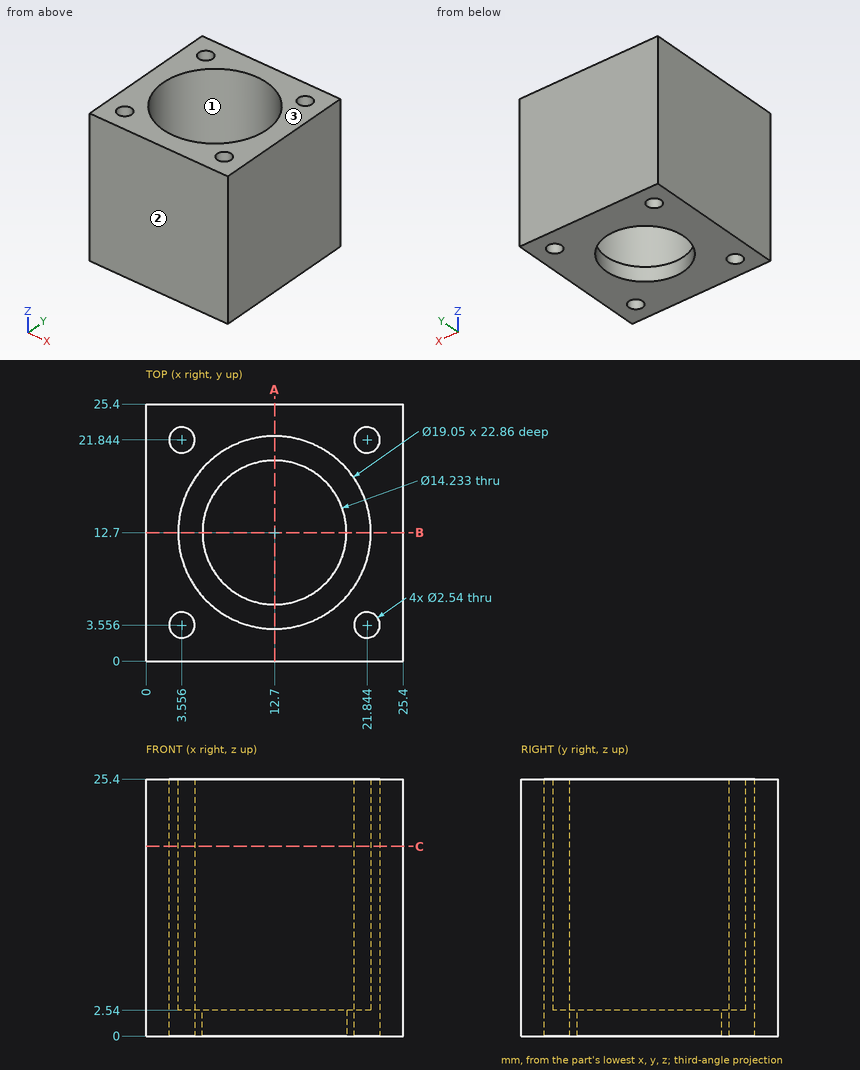
Check sheet for the drawn part. Datum: minimum x, y, z corner. Units: mm. Round coordinates to 2 decimals unless told otherwise and drop trailing zeros. Order: outer loops, then holes, each group sorted by start corner. A loop starts at its lowest first (then second) coordinate and runs counter-clockwise, first axis right, second up.
(1) Cross-section at A-A, the plane x = 12.7. Enter the section's corners in (y, z) (1 decimal).
(2) Draft check along Y on the marked faces 1, 2 and 3. Enter one of: pulls with the +Y half, pulls with the -Y half, needs draft (parallel to the pull), parting line crosses it, or undercut.
(3) Scan lines: probe 1 along X at (y, z) = (20.75, 18.5); probe 2 along Y at (x, z) = (12.7, 7.5) (3 decimals); probe 3 along Y at (x, z) = (21, 17.5) (3 decimals). Record each from-to range of solid material in increasing order.
(4) Cross-section at C-C, the plane z = 18.75. Enter the section's corners in (x, y) (3 decimals), and give its area (3 significant figures).
(5) Go/stop test with flat-tipped pins: P1, Ø15, axis at x = 12.7, y = 12.7, coming from the +Z side; P2, Ø1.5, axis at x = 3.556, y = 3.556, coming from the -Z side. Record where each tip stops, or that it passes through.
Check sheet entries:
1. outline: (0, 0) - (5.6, 0) - (5.6, 2.5) - (3.2, 2.5) - (3.2, 25.4) - (0, 25.4) - close; (19.8, 0) - (25.4, 0) - (25.4, 25.4) - (22.2, 25.4) - (22.2, 2.5) - (19.8, 2.5) - close
2. face 1: undercut
2. face 2: pulls with the -Y half
2. face 3: needs draft
3. probe 1: x = 0 to 2.91, 4.2 to 7.61, 17.79 to 21.2, 22.49 to 25.4
3. probe 2: y = 0 to 3.175, 22.225 to 25.4
3. probe 3: y = 0 to 2.607, 4.505 to 8.027, 17.373 to 20.895, 22.793 to 25.4
4. outline: (0, 0) - (25.4, 0) - (25.4, 25.4) - (0, 25.4) - close; hole circle Ø2.54 at (3.556, 3.556); hole circle Ø2.54 at (3.556, 21.844); hole circle Ø19.05 at (12.7, 12.7); hole circle Ø2.54 at (21.844, 3.556); hole circle Ø2.54 at (21.844, 21.844)
4. area: 340 mm2
5. P1: stops at z = 2.54
5. P2: passes through
